Can you work these out from the model? Positions are in its coordinate system, mm. A direction names the side the tool comes from. Round coordinates to 2 decimals unless told otherwise and drop trailing zeros. Write each loop counter-clockwise with the first axis right and the second up, starting at its lowest first coordinate (ties: lowest second). Pieces come first, ordered by that corner, then holes. Notation, with made-up numbers: M 43.25,8.25 L 97.25,8.25 A20 ccw 97.25,22.25 Z; hole C 86,-22.75 d8. An arc over 180 degrees is marked long. Answer in a Markdown table with one row per item. Add a question column.
(1) Suppose I cut it at B-B, the plane y = 6.75. Write out the boundary of the cut face in (x, z), then the cut area to 3 significant figures.
(2) For faces 1 (the face through (10, 1, 0)), 2 (the face through (11, 28.4, 15)), 3 (the face through (14, 6, 2)), 4 (the face through (-1, 16, -15)), 5 (the face through (0, 3, 0)), which set-ups out of +Z, -Z, +X, -X, +Y, -Y let a thin tool reach every point of the face, with its end or its side?
(3) I'm going to push flat-ended pins straight in: pin 1 (6.5 mm diameter, centred on x = -12.5, z = 1, fed in from -Y); pin 2 (15.5 mm diameter, centred on x = -15, y = 17.5, fed in from +Z); pin 3 (0.9 mm diameter, centred on y = 15.5, z = 15, fed in from -X); pin 4 (4 mm diameter, centred on x = 14, z = -1, fed in from +Y). Where does each tip first touch, or does it pass through?
(4) Suppose I cut it at A-A, the plane x = -13. Write out the boundary of the cut face in (y, z), then the cut area to 3 significant figures.
(5) Suppose I cut it at C-C, the plane z = 0. Write out the boundary of the cut face in (x, y), then the cut area to 3 significant figures.
(6) If we mould it in two halves opening along X, with no side actions, what happens to faces 6 (the face through (-11, 3, -1)), 7 (the face through (-11, 28.4, -15)), 8 (the face through (1, 16, 15)), 9 (the face through (15, 3, -1))? For each: released by +X, released by -X, zero draft, split by the parting line, or undercut.
(7) If I drill on probe 1 along Z at (x, y) = (-13, 1.3); probe 2 along Z at (x, y) = (13, 5.4); probe 3 along Z at (x, y) = (-13, 5.1), over which ranges is the centre line in solid material (lowest first)?
(8) Suppose I cut it at D-D, the plane x = -5. Write out the boundary of the cut face in (y, z), then the cut area to 3 significant figures.
Autodesk Inventor part; units mm, degrees
ref_plane "YZ Plane" through (0, 0, 0) normal (1, 0, 0) x (0, 1, 0)
ref_plane "XZ Plane" through (0, 0, 0) normal (0, 1, 0) x (-1, 0, 0)
ref_plane "XY Plane" through (0, 0, 0) normal (0, 0, 1) x (1, 0, 0)
sketch "Sketch1" plane through (0, 0, 0) normal (0, 1, 0) x (-1, 0, 0)
  line L0 (20.5, 16.2) -> (-20.5, 16.2)
  line L1 (-20.5, 16.2) -> (-20.5, -16.2)
  line L2 (-20.5, -16.2) -> (20.5, -16.2)
  line L3 (20.5, -16.2) -> (20.5, 16.2)
  point P0 (0, 0)
  dimension "d0" = 41
  dimension "d1" = 32.4
extrude "Extrusion1" add sketch "Sketch1" along normal blind 3
sketch "Sketch3" plane through (0, 3, 0) normal (0, 1, 0) x (1, 0, 0)
  line L0 (-20.5, -16.2) -> (20.5, -16.2)
  line L1 (-20.5, 16.2) -> (-20.5, -16.2)
  line L2 (20.5, -16.2) -> (-20.5, -16.2)
  line L3 (-20.5, -16.2) -> (-20.5, -13.2)
  line L4 (-20.5, -13.2) -> (20.5, -13.2)
  line L5 (20.5, -13.2) -> (20.5, -16.2)
  line L6 (20.5, 16.2) -> (-20.5, 16.2)
  line L7 (20.5, 16.2) -> (-20.5, 16.2)
  line L8 (-20.5, 16.2) -> (-20.5, 13.2)
  line L9 (-20.5, 13.2) -> (20.5, 13.2)
  line L10 (20.5, 13.2) -> (20.5, 16.2)
  point P0 (0, 0)
  dimension "d8" = 3
  dimension "d9" = 3
extrude "Extrusion3" add sketch "Sketch3" along normal blind 25.4
sketch "Sketch4" plane through (20.5, 0, -16.2) normal (0, 0, -1) x (-1, 0, 0)
  line L0 (41, 3) -> (0, 3)
  line L1 (0, 28.4) -> (41, 28.4)
  line L2 (0, 3) -> (21.5, 3)
  line L3 (21.5, 3) -> (21.5, 28.4)
  line L4 (21.5, 28.4) -> (0, 28.4)
  line L5 (0, 28.4) -> (0, 3)
  point P0 (20.5, 0)
  dimension "d12" = 21.5
extrude "Extrusion4" cut sketch "Sketch4" against normal blind 3
sketch "Sketch5" plane through (-20.5, 0, 16.2) normal (0, 0, 1) x (1, 0, 0)
  line L0 (41, 28.4) -> (0, 28.4)
  line L1 (19.5, 3) -> (41, 3)
  line L2 (0, 28.4) -> (21.5, 28.4)
  line L3 (21.5, 28.4) -> (21.5, 3)
  line L4 (21.5, 3) -> (0, 3)
  line L5 (0, 3) -> (0, 28.4)
  point P0 (20.5, 0)
  dimension "d15" = 21.5
extrude "Extrusion5" cut sketch "Sketch5" against normal blind 3
sketch "Sketch6" plane through (0, 3, 0) normal (0, 1, 0) x (1, 0, 0)
  circle A0 centre (13, 0) radius 4.25
  circle A1 centre (-13, 0) radius 4.25
  point P0 (0, 0)
  dimension "d20" = 8.5
  dimension "d21" = 8.5
extrude "Extrusion6" add sketch "Sketch6" along normal blind 3
sketch "Sketch7" plane through (0, 0, 0) normal (0, -1, 0) x (1, 0, 0)
  circle A0 centre (-13, 0) radius 4.25
  circle A1 centre (-13, 0) radius 2
  circle A2 centre (13, 0) radius 4.25
  circle A3 centre (13, 0) radius 2
  point P0 (0, 0)
  dimension "d24" = 4
  dimension "d25" = 4
extrude "Extrusion7" cut sketch "Sketch7" against normal blind 6 contours A1 | A3
sketch "Sketch8" plane through (0, 0, 0) normal (0, -1, 0) x (1, 0, 0)
  circle A0 centre (-13, 0) radius 2
  circle A1 centre (-13, 0) radius 3
  circle A2 centre (13, 0) radius 2
  circle A3 centre (13, 0) radius 3
  point P0 (0, 0)
  dimension "d28" = 6
  dimension "d29" = 6
extrude "Extrusion8" cut sketch "Sketch8" against normal blind 3 contours A0 | A1 | A2 | A3
properties part number "stepperBracket"
Calculated:
| question | item | result |
|---|---|---|
| 1 | outline | M -20.5,-16.2 L -1,-16.2 L -1,-13.2 L -20.5,-13.2 Z; M 1,13.2 L 20.5,13.2 L 20.5,16.2 L 1,16.2 Z |
| 1 | area | 117 mm² |
| 2 | face 1 | -Y |
| 2 | face 2 | +Z, -Z, +X, -X, +Y |
| 2 | face 3 | -Z, +X, -X, +Y |
| 2 | face 4 | +Z, -Z, +X, +Y |
| 2 | face 5 | +Y |
| 3 | pin 1 | y = 0 |
| 3 | pin 2 | z = -13.2 |
| 3 | pin 3 | x = 1 |
| 3 | pin 4 | y = 6 |
| 4 | outline | M 0,-16.2 L 28.4,-16.2 L 28.4,-13.2 L 3,-13.2 L 3,-4.25 L 6,-4.25 L 6,-2 L 3,-2 L 3,-3 L 0,-3 Z; M 0,3 L 3,3 L 3,2 L 6,2 L 6,4.25 L 3,4.25 L 3,16.2 L 0,16.2 Z |
| 4 | area | 169 mm² |
| 5 | outline | M -20.5,0 L -16,0 L -16,3 L -15,3 L -15,6 L -17.25,6 L -17.25,3 L -20.5,3 Z; M -11,3 L -10,3 L -10,0 L 10,0 L 10,3 L 11,3 L 11,6 L 8.75,6 L 8.75,3 L -8.75,3 L -8.75,6 L -11,6 Z; M 15,3 L 16,3 L 16,0 L 20.5,0 L 20.5,3 L 17.25,3 L 17.25,6 L 15,6 Z |
| 5 | area | 114 mm² |
| 6 | face 6 | undercut |
| 6 | face 7 | zero draft |
| 6 | face 8 | released by -X |
| 6 | face 9 | undercut |
| 7 | probe 1 | -16.2 to -3, 3 to 16.2 |
| 7 | probe 2 | -4.25 to -2, 2 to 4.25, 13.2 to 16.2 |
| 7 | probe 3 | -16.2 to -13.2, -4.25 to -2, 2 to 4.25 |
| 8 | outline | M 0,-16.2 L 28.4,-16.2 L 28.4,-13.2 L 3,-13.2 L 3,16.2 L 0,16.2 Z |
| 8 | area | 173 mm² |
